The model under review builds one solid part; all positions refer to its coordinate system, in mm. Face numbers are marked on the shaded views. A direction names the side the tool comes from. Coordinates: 2 decimals unless noted, no trailing zeros. Loops run counter-clockwise (first coordinate to the right, second up) from the corner with the lowest first, then second, coordinate; pieces in that order, holes last. Notation, with made-up numbers: M 42.25,72 L 97.25,72 A20 ccw 97.25,94 Z; hole C -15.5,-18 d6. An arc over 180 degrees is marked long. Use one line per item in the form item = value.
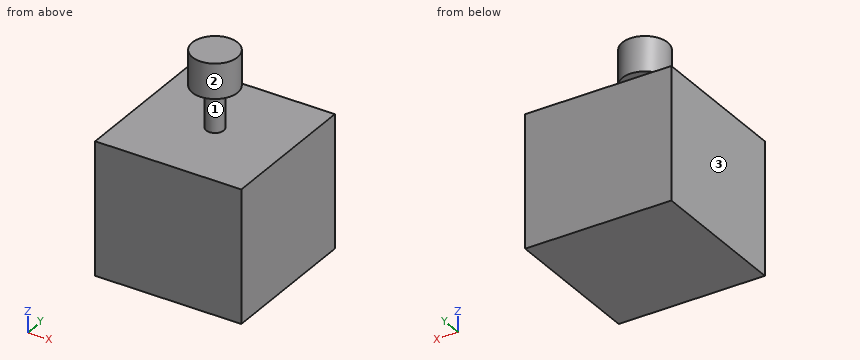
```python
from build123d import *

# Parameters (mm, degrees)
SKETCH1_W           = 42
SKETCH1_H           = 42
BOSS_EXTRUDE1_DEPTH = 38
SKETCH2_R           = 2.5
BOSS_EXTRUDE2_DEPTH = 22
SKETCH3_R           = 6.5
BOSS_EXTRUDE3_DEPTH = 10


with BuildPart() as part:
    # Sketch1 → Boss-Extrude1 (new body)
    with BuildSketch(Plane.XY):
        Rectangle(SKETCH1_W, SKETCH1_H)
    extrude(amount=BOSS_EXTRUDE1_DEPTH)

    # Sketch2 → Boss-Extrude2 (add)
    with BuildSketch(Plane.XY.offset(38)):
        Circle(SKETCH2_R)
    extrude(amount=BOSS_EXTRUDE2_DEPTH)

    # Sketch3 → Boss-Extrude3 (add)
    with BuildSketch(Plane.XY.offset(60)):
        Circle(SKETCH3_R)
    extrude(amount=-BOSS_EXTRUDE3_DEPTH)


solid = part.part
```
1. Wall thickness on line 1 along Z through (x, y) = (5.5, 2); line 2 along Z through (x, y) = (8.5, 17.5); line 3 along X through (y, z) = (1, 38.5): over which ranges is each line inside the solid? List them lowest first. Write a range as from..to.
Response values:
line_1 = 0..38, 50..60
line_2 = 0..38
line_3 = -2.29..2.29
2. Add section D-D (z = 43). State the section outline as (x, y) points, then the cut area to 3 significant figures.
Response values:
outline = C 0,0 d5
area = 19.6 mm^2
3. Machinability: for the marked faces 1, 2 and 3, which of the approach directions +Z, -Z, +X, -X, +Y, -Y give a long, thin tool a straight path to every point of the face, cutting with its end or side? Answer none if there is none.
Response values:
face_1 = none
face_2 = +Z
face_3 = +Z, -Z, -X, +Y, -Y
4. Insertion check: P1, Ø6, axis at x = -15.5, y = 3.5, coming from the -Z side; P2, Ø6, axis at x = 0, z = 48.5, coming from the +Y side; P3, Ø12, axis at x = 15, z = 46, coming from the -Y side; P4, Ø1.5, axis at x = -15, y = 14, coming from the +Z side. Each pin has a flat end and moves straight along its axis. Give the tip position at first contact, or say it passes through.
Response values:
P1 = 0
P2 = 6.5
P3 = through
P4 = 38
5. Add section C-C (y = -4.5). State the section outline as (x, z) points, then the cut area to 3 significant figures.
Response values:
outline = M -21,0 L 21,0 L 21,38 L -21,38 Z; M -4.69,50 L 4.69,50 L 4.69,60 L -4.69,60 Z
area = 1,690 mm^2
6. Add section A-A (x = 0). State the section outline as (y, z) points, then the cut area to 3 significant figures.
Response values:
outline = M -21,0 L 21,0 L 21,38 L 2.5,38 L 2.5,50 L 6.5,50 L 6.5,60 L -6.5,60 L -6.5,50 L -2.5,50 L -2.5,38 L -21,38 Z
area = 1,790 mm^2
